Solid Edge part; units mm, degrees
sketch "Sketch1" plane through (0, 0, 0) normal (1, 0, 0) x (0, 1, 0)
  line L0 (79.375, 19.05) -> (0, 19.05)
  line L1 (0, 19.05) -> (0, 0)
  line L2 (0, 0) -> (79.375, 0)
  line L3 (79.375, 0) -> (79.375, 19.05)
extrude "Protrusion1" add sketch "Sketch1" along normal blind 114.3
shell "Thinwall_1" thickness 3.175 removed faces 3 at (114.3, 65.3521, 2.9845) at (94.107, 0, 16.0655) at (0, 65.3521, 2.9845)
sketch "Sketch2" plane through (0, 0, 0) normal (1, 0, 0) x (0, 1, 0)
  line L0 (79.375, 184.15) -> (79.375, 19.05)
  line L1 (79.375, 19.05) -> (66.675, 19.05)
  line L2 (66.675, 19.05) -> (66.675, 184.15)
  line L3 (66.675, 184.15) -> (79.375, 184.15)
extrude "Protrusion2" add sketch "Sketch2" along normal up to vertex (114.3 mm away)
properties material "ABS Plastic, medium impact"
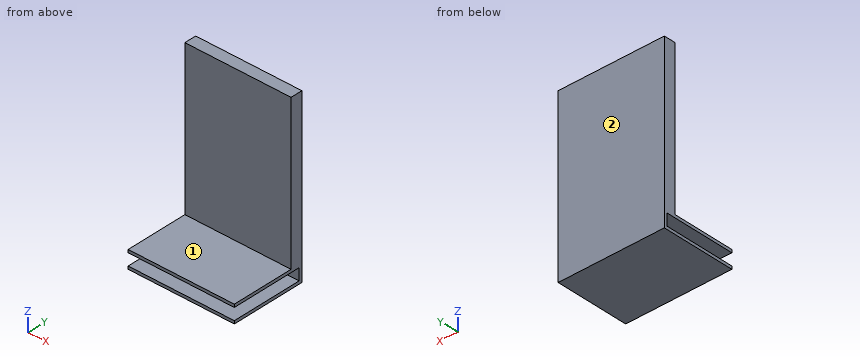
For this review, take the finished solid that the model builds, in its own axes (mm). Face numbers are marked on the shaded views. A direction names the side the tool comes from. Give positions to 0.01 mm unless a question says otherwise; leave off trailing zeros. Write each loop counter-clockwise with the first axis right and the second up, starting at its lowest first coordinate (ties: lowest second). Pieces come first, ordered by that corner, then holes. Notation, with made-up numbers: M -26.75,45 L 18.25,45 A27 cw 18.25,63 Z; hole C 11.25,-22 d1. An arc over 180 degrees is marked long. Answer as a JSON object with one key per item and string values. Group by question number.
Item 1: Tool access review of the marked faces 1 and 2: name each direction out of +Z, -Z, +X, -X, +Y, -Y from which nothing blocks a thin tool from reaching the whole face with its end or side.
Item 2: For probe 1 along Z at (x, y) = (99, 48) (3 decimals); probe 2 along Y at (x, z) = (35, 117) (3 decimals); probe 3 along Y at (x, z) = (70.5, 8) (3 decimals), list the stretches that pass through material, from the lowest coordinate up. Write a range as [from, to].
Item 3: Consider section B-B on x = 34. Write out the cut boundary in (y, z) (3 decimals), plus the area to 3 significant figures.
Item 4: Consider section D-D on y = 69. Write out the cut boundary in (x, z) (3 decimals), plus the area to 3 significant figures.
Item 5: For pin 1 Ø3 at (x, z) = (29.5, 40.5) entering from -Y (3 decimals); pin 2 Ø4 at (x, y) = (69, 15.5) entering from +Z, all flat-tipped, find the tip position at first contact; note any pin that passes through.
Item 6: Consider section C-C on z = 110.5. Write out the cut boundary in (x, y) (3 decimals).
Item 7: Consider section A-A on y = 51.5. Write out the cut boundary in (x, z) (3 decimals), plus the area to 3 significant figures.
Check result:
{
 "1": {"face 1": "+Z, +X, -X, -Y", "face 2": "+Z, -Z, +X, -X, +Y"},
 "2": {"probe 1": "z = [0, 3.175], [15.875, 19.05]", "probe 2": "y = [66.675, 79.375]", "probe 3": "y = [76.2, 79.375]"},
 "3": {"outline": "M 0,0 L 79.375,0 L 79.375,184.15 L 66.675,184.15 L 66.675,19.05 L 0,19.05 L 0,15.875 L 76.2,15.875 L 76.2,3.175 L 0,3.175 Z", "area": "2,640 mm^2"},
 "4": {"outline": "M 0,0 L 114.3,0 L 114.3,3.175 L 0,3.175 Z; M 0,15.875 L 114.3,15.875 L 114.3,184.15 L 0,184.15 Z", "area": "19,600 mm^2"},
 "5": {"pin 1": "stops at y = 66.675", "pin 2": "stops at z = 19.05"},
 "6": {"outline": "M 0,66.675 L 114.3,66.675 L 114.3,79.375 L 0,79.375 Z"},
 "7": {"outline": "M 0,0 L 114.3,0 L 114.3,3.175 L 0,3.175 Z; M 0,15.875 L 114.3,15.875 L 114.3,19.05 L 0,19.05 Z", "area": "726 mm^2"}
}
